from build123d import *

# Parameters (mm, degrees)
SKETCH1_W           = 330
SKETCH1_H           = 45
BOSS_EXTRUDE1_DEPTH = 33
SKETCH2_R           = 20
CUT_EXTRUDE1_DEPTH  = 40
SKETCH3_W           = 19
SKETCH3_H           = 31
CUT_EXTRUDE2_DEPTH  = 260


with BuildPart() as part:
    # Sketch1 → Boss-Extrude1 (new body)
    with BuildSketch(Plane.XY):
        Rectangle(SKETCH1_W, SKETCH1_H)
    extrude(amount=BOSS_EXTRUDE1_DEPTH)

    # Sketch2 → Cut-Extrude1 (cut)
    with BuildSketch(Plane.XY.offset(33)):
        with Locations((-135, 0)):
            Circle(SKETCH2_R)
        with BuildLine():
            Line((-135, 22.5), (-173.521075779, 35.069593385))
            Line((-173.521075779, 35.069593385), (-171.569663812, -40.136425611))
            Line((-171.569663812, -40.136425611), (-135, -22.5))
            ThreePointArc((-135, -22.5), (-157.5, 0), (-135, 22.5))
        make_face()
    extrude(amount=-CUT_EXTRUDE1_DEPTH, mode=Mode.SUBTRACT)

    # Sketch3 → Cut-Extrude2 (cut)
    with BuildSketch(Plane(origin=(165, 0, 0), x_dir=(0, 0, -1), z_dir=(1, 0, 0))):
        with Locations((-16.5, 0)):
            Rectangle(SKETCH3_W, SKETCH3_H)
    extrude(amount=-CUT_EXTRUDE2_DEPTH, mode=Mode.SUBTRACT)


solid = part.part
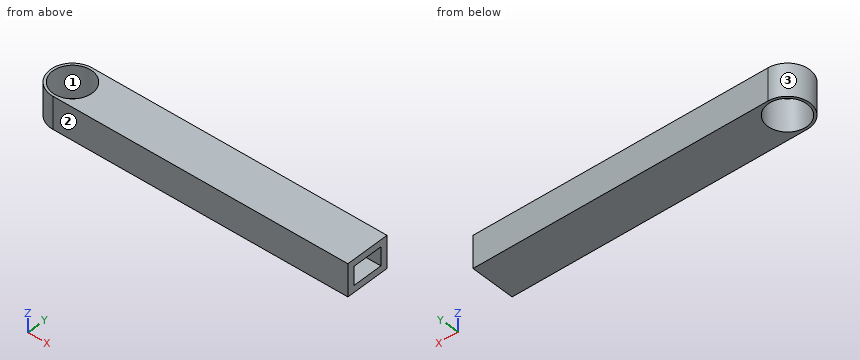
Verification items for the finished model (mm, model axes). Face numbers are marked on the shaded views. Give positions to 0.01 mm unless a question says otherwise; leave off trailing zeros. Write each loop counter-clockwise with the first axis right and the second up, starting at its lowest first coordinate (ties: lowest second). Pieces come first, ordered by that corner, then holes. Notation, with made-up numbers: (-27.75, -9) -> (-12.75, -9) arc R37 cw to (-12.75, 27) -> close; hole circle Ø1 at (75, 14.25). An arc over 180 degrees is marked (long way). Use CSV: the item, a comma, the result in double quotes.
(1) Sectioned sample at C-C (x = 35). Record the cut outline in (y, z).
Derived:
outline,"(-22.5, 0) -> (22.5, 0) -> (22.5, 33) -> (-22.5, 33) -> close; hole (-15.5, 7) -> (15.5, 7) -> (15.5, 26) -> (-15.5, 26) -> close"
(2) Sectioned sample at D-D (y = -12.5). Record the cut outline in (x, z), plus the area to 3 significant figures.
Derived:
outline,"(-153.71, 0) -> (-150.61, 0) -> (-150.61, 33) -> (-153.71, 33) -> close; (-119.39, 0) -> (165, 0) -> (165, 7) -> (-95, 7) -> (-95, 26) -> (165, 26) -> (165, 33) -> (-119.39, 33) -> close"
area,"4,550 mm^2"
(3) Go/stop test with a flat-tipped pin: pin 1 (24 mm diameter, centred on x = -135, y = 0, fed in from +Z). Record where the tip stops, or that it passes through.
Derived:
pin 1,"passes through"
(4) Release check for a two-part mould opening along X. For the marked faces 1, 2 and 3 record: +X half, -X half, draft (parallel to the pull), parting line (faces both ways), or undercut.
Derived:
face 1,"undercut"
face 2,"draft"
face 3,"-X half"
(5) Sectioned sample at A-A (y = 3.5). Record the cut outline in (x, z), plus the area to 3 significant figures.
Derived:
outline,"(-157.23, 0) -> (-154.69, 0) -> (-154.69, 33) -> (-157.23, 33) -> close; (-115.31, 0) -> (165, 0) -> (165, 7) -> (-95, 7) -> (-95, 26) -> (165, 26) -> (165, 33) -> (-115.31, 33) -> close"
area,"4,390 mm^2"
(6) Material ranges on L1, parallel to Z at x = 128, y = 9; L2, parallel to Y at x = -135, z = 14; L3, parallel to X at y = -1, z = 25.5, recorded low to high.
Derived:
L1,"z = 0 to 7, 26 to 33"
L2,"y = -22.5 to -20, 20 to 22.5"
L3,"x = -157.48 to -154.97, -115.03 to -95"
(7) Sectioned sample at B-B (z = 11.5). Record the cut outline in (x, y), plus the area to 3 significant figures.
Derived:
outline,"(-135, -22.5) -> (165, -22.5) -> (165, -15.5) -> (-95, -15.5) -> (-95, 15.5) -> (165, 15.5) -> (165, 22.5) -> (-135, 22.5) arc R22.5 ccw to start; hole circle Ø40 at (-135, 0)"
area,"4,980 mm^2"
